from build123d import *

# Parameters (mm, degrees)
F0_R     = 3.96875
F0_R_2   = 1.7272
F1_DEPTH = 3.175


with BuildPart() as f1:
    # F0 (on Top) → F1 (new body)
    with BuildSketch(Plane.XY):
        with BuildLine():
            Line((31.75, 28.964184), (22.225, 28.964184))
            Line((22.225, 28.964184), (-5.752253, 21.467701))
            ThreePointArc((-5.752253, 21.467701), (-22.225, 0), (-5.752253, -21.467701))
            Line((-5.752253, -21.467701), (22.225, -28.964184))
            Line((22.225, -28.964184), (31.75, -28.964184))
            Line((31.75, -28.964184), (31.75, 28.964184))
        make_face()
        with Locations((-11.786586, -11.786586)):
            Circle(F0_R, mode=Mode.SUBTRACT)
        with Locations((11.786586, -11.786586)):
            Circle(F0_R_2, mode=Mode.SUBTRACT)
        with Locations((-11.786586, 11.786586)):
            Circle(F0_R_2, mode=Mode.SUBTRACT)
        Circle(F0_R, mode=Mode.SUBTRACT)
        with Locations((11.786586, 11.786586)):
            Circle(F0_R, mode=Mode.SUBTRACT)
    extrude(amount=F1_DEPTH)


solid = f1.part
Input: part model. Units: mm. Frame: model coordinates. Coordinates: 2 decimals unless noted, no trailing zeros. Loops run counter-clockwise (first coordinate to the right, second up) from the corner with the lowest first, then second, coordinate; pieces in that order, holes last.
(1) Section A-A on y = 0. Return the cut outline in (x, z) (3 decimals), then the cut area to 3 significant figures.
(2) Section D-D on y = -6.5. Return the cut outline in (x, z) (3 decimals).
(3) Material intervals for probe 1 along Y at (x, z) = (-11, 0.35); probe 2 along Y at (x, z) = (-11.5, 2.9); probe 3 along X at (y, z) = (14, 1.15), sorted ascending.
(4) Section C-C on z = 1.7. Count the separate pieces of the cut face and the enclosed holes in it, then the cut area to 3 significant figures.
(5) Pull-direction query (Y, two-part tool) for faces 1 (the face through (-12.65, -15.66, 1.57)), 2 (the face through (27, -28.964, 2)), 3 (the face through (-22.22, 0.41, 1.57)); classes: released by +Y, released by -Y, zero draft, split by the parting line, or undercut.
(6) Section B-B on x = 0. Return the cut outline in (y, z) (3 decimals).
Data:
1. outline: (-22.225, 0) - (-3.969, 0) - (-3.969, 3.175) - (-22.225, 3.175) - close; (3.969, 0) - (31.75, 0) - (31.75, 3.175) - (3.969, 3.175) - close
1. area: 146 mm2
2. outline: (-21.253, 0) - (31.75, 0) - (31.75, 3.175) - (-21.253, 3.175) - close
3. probe 1: y = -19.31 to -15.68, -7.9 to 10.25, 13.32 to 19.31
3. probe 2: y = -19.02 to -15.74, -7.83 to 10.08, 13.49 to 19.02
3. probe 3: x = -17.26 to 8.49, 15.08 to 31.75
4. separate pieces: 1
4. enclosed holes: 5
4. area: 2,320 mm2
5. face 1: undercut
5. face 2: released by -Y
5. face 3: split by the parting line
6. outline: (-23.009, 0) - (-3.969, 0) - (-3.969, 3.175) - (-23.009, 3.175) - close; (3.969, 0) - (23.009, 0) - (23.009, 3.175) - (3.969, 3.175) - close
